Read the model definition and answer for the solid it produces. Units are mm, in the model's axes. A direction names the side the tool comes from. Give positions to 0.01 mm unless a question says otherwise; leave off trailing zeros. Write each loop counter-clockwise with the first axis right and the second up, starting at its lowest first coordinate (ties: lowest second). Pieces come first, ordered by that corner, then holes. Notation, with made-up numbers: (85.5, 20.5) - (131.5, 20.5) arc R31 ccw to (131.5, 44.5) - close; hole circle Ø5 at (-12.75, -18.75). An arc over 180 degrees is marked (long way). Use CSV: the item, a comma, the result in double quotes. Start each with the question number.
from build123d import *

# Parameters (mm, degrees)
SKETCH1_R           = 65
SKETCH1_R_2         = 3
SKETCH1_R_3         = 1.5
SKETCH1_R_4         = 2.5
SKETCH1_R_5         = 9.5
BOSS_EXTRUDE1_DEPTH = 10
SKETCH1_3_R         = 9.5
BOSS_EXTRUDE2_DEPTH = 5
SKETCH2_R           = 5
CUT_EXTRUDE1_DEPTH  = 5
SKETCH3_R           = 2.5
CUT_EXTRUDE2_DEPTH  = 10
SKETCH4_R           = 5
CUT_EXTRUDE3_DEPTH  = 5


with BuildPart() as part:
    # Sketch1 → Boss-Extrude1 (new body)
    with BuildSketch(Plane(origin=(0, 0, 0), x_dir=(1, 0, 0), z_dir=(0, 1, 0))):
        with Locations(Location((0, 0, 0), (0, 0, 270))):
            Circle(SKETCH1_R)
        with Locations(Location((0, 0, 0), (0, 0, 270))):
            Circle(SKETCH1_R_2, mode=Mode.SUBTRACT)
        with Locations(Location((0, 9.5, 0), (0, 0, 270))):
            Circle(SKETCH1_R_3, mode=Mode.SUBTRACT)
        with Locations(Location((8.227241336, 4.75, 0), (0, 0, 270))):
            Circle(SKETCH1_R_3, mode=Mode.SUBTRACT)
        with Locations(Location((8.227241336, -4.75, 0), (0, 0, 270))):
            Circle(SKETCH1_R_3, mode=Mode.SUBTRACT)
        with Locations(Location((0, -9.5, 0), (0, 0, 270))):
            Circle(SKETCH1_R_3, mode=Mode.SUBTRACT)
        with Locations(Location((-8.227241336, -4.75, 0), (0, 0, 270))):
            Circle(SKETCH1_R_3, mode=Mode.SUBTRACT)
        with Locations(Location((-8.227241336, 4.75, 0), (0, 0, 270))):
            Circle(SKETCH1_R_3, mode=Mode.SUBTRACT)
        with Locations(Location((0, -60, 0), (0, 0, 270))):
            Circle(SKETCH1_R_4, mode=Mode.SUBTRACT)
        with Locations(Location((-60, 0, 0), (0, 0, 270))):
            Circle(SKETCH1_R_4, mode=Mode.SUBTRACT)
        with Locations(Location((0, 60, 0), (0, 0, 270))):
            Circle(SKETCH1_R_4, mode=Mode.SUBTRACT)
        with Locations(Location((20, 0, 0), (0, 0, 270))):
            Circle(SKETCH1_R_5, mode=Mode.SUBTRACT)
        with Locations(Location((-3.048738704, 32.260845552, 0), (0, 0, 270))):
            Circle(SKETCH1_R_3, mode=Mode.SUBTRACT)
        with Locations(Location((30.001268663, 32.260845552, 0), (0, 0, 270))):
            Circle(SKETCH1_R_3, mode=Mode.SUBTRACT)
        with Locations(Location((55.001268663, 0.260845552, 0), (0, 0, 270))):
            Circle(SKETCH1_R_4, mode=Mode.SUBTRACT)
        with Locations(Location((30.001268663, -31.739154448, 0), (0, 0, 270))):
            Circle(SKETCH1_R_3, mode=Mode.SUBTRACT)
        with Locations(Location((-3.048738704, -31.739154448, 0), (0, 0, 270))):
            Circle(SKETCH1_R_3, mode=Mode.SUBTRACT)
    extrude(amount=BOSS_EXTRUDE1_DEPTH)

    # Sketch1<3> → Boss-Extrude2 (add)
    with BuildSketch(Plane(origin=(0, 0, 0), x_dir=(1, 0, 0), z_dir=(0, 1, 0))):
        with Locations(Location((20, 0, 0), (0, 0, 270))):
            Circle(SKETCH1_3_R)
    extrude(amount=BOSS_EXTRUDE2_DEPTH)

    # Sketch2 → Cut-Extrude1 (cut)
    with BuildSketch(Plane.XZ):
        with Locations(Location((30.001268663, 31.739154448, 0), (0, 0, 270))):
            Circle(SKETCH2_R)
        with Locations(Location((-3.048738704, 31.739154448, 0), (0, 0, 270))):
            Circle(SKETCH2_R)
        with Locations(Location((55.001268663, -0.260845552, 0), (0, 0, 270))):
            Circle(SKETCH2_R)
        with Locations(Location((30.001268663, -32.260845552, 0), (0, 0, 270))):
            Circle(SKETCH2_R)
        with Locations(Location((-3.048738704, -32.260845552, 0), (0, 0, 270))):
            Circle(SKETCH2_R)
    extrude(amount=-CUT_EXTRUDE1_DEPTH, mode=Mode.SUBTRACT)

    # Sketch3 → Cut-Extrude2 (cut)
    with BuildSketch(Plane(origin=(0, 10, 0), x_dir=(1, 0, 0), z_dir=(0, 1, 0))):
        with Locations(Location((-48.498731337, 0.260845552, 0), (0, 0, 270))):
            Circle(SKETCH3_R)
    extrude(amount=-CUT_EXTRUDE2_DEPTH, mode=Mode.SUBTRACT)

    # Sketch4 → Cut-Extrude3 (cut)
    with BuildSketch(Plane.XZ):
        with Locations(Location((-48.498731337, -0.260845552, 0), (0, 0, 270))):
            Circle(SKETCH4_R)
    extrude(amount=-CUT_EXTRUDE3_DEPTH, mode=Mode.SUBTRACT)


solid = part.part
(1) The part is cut by section A-A on z = -60. Write down the section's boundary in (x, y), plus the area to 3 significant figures.
(2) The part is cut by section C-C on y = 6.5. Give the number of separate pieces and of enclosed holes in the cut face, plus the area to 3 significant figures.
(3) Which of the six approach directions +Z, -Z, +X, -X, +Y, -Y give full straight-line access (tool end or side, diameter ignored) to faces 1 (the face through (30.45, 7.46, -30.83)), 2 (the face through (26.96, 2.46, 35.71))?
(4) For a pull along Z with two mould halves and no side action, classify faces 3 (the face through (-14, 0, -1)), 4 (the face through (-6.962, 4.93, 5.556)), 5 (the face through (0.9, 4.93, 2.86)) as pulls with the +Z half, pulls with the -Z half, needs draft (parallel to the pull), parting line crosses it, or undercut.
(5) The part is cut by section B-B on x = -60. Write down the section's boundary in (y, z), plus the area to 3 significant figures.
(6) Consider probe 1 along X at (y, z) = (6, 0); probe 2 along X at (y, z) = (1.75, -34.5); probe 3 along Z at (x, y) = (-2, 1.5). Determine where each line is inside the solid, lowest interval first.
(7) Given P1, Ø3, axis at y = 6, z = -15, coming from the +X side; P2, Ø2.5, axis at x = -3.05, z = 31.74, coming from the -Y side; P3, Ø6, axis at x = 46.5, y = 6, coming from the +Z side; P4, Ø4, axis at y = 6, z = 45.5, coming from the -X side, each flat-ended and moving along its own axis, determine where each tip first touches the part or whether it passes through.
Reported:
1,outline,"(-25, 0) - (-2.5, 0) - (-2.5, 10) - (-25, 10) - close; (2.5, 0) - (25, 0) - (25, 10) - (2.5, 10) - close"
1,area,"450 mm²"
2,separate pieces,"1"
2,enclosed holes,"17"
2,area,"12,800 mm²"
3,face 1,"+Y, -Y"
3,face 2,"-Y"
4,face 3,"needs draft"
4,face 4,"undercut"
4,face 5,"undercut"
5,outline,"(0, -25) - (10, -25) - (10, -2.5) - (0, -2.5) - close; (0, 2.5) - (10, 2.5) - (10, 25) - (0, 25) - close"
5,area,"450 mm²"
6,probe 1,"-65 to -62.5, -57.5 to -50.99, -46.01 to -3, 3 to 10.5, 29.5 to 52.51, 57.49 to 65"
6,probe 2,"-55.09 to -7.52, 1.42 to 25.53, 34.47 to 55.09"
6,probe 3,"-64.97 to -61.5, -58.5 to -37.15, -27.37 to -2.24, 2.24 to 26.85, 36.63 to 58.5, 61.5 to 64.97"
7,P1,"x = 63.58"
7,P2,"through"
7,P3,"z = 48.3"
7,P4,"x = -48.3"
